from build123d import *

# Parameters (mm, degrees)
BOSS_EXTRUDE1_DEPTH = 20
CUT_EXTRUDE1_DEPTH  = 17
SKETCH3_R           = 2
BOSS_EXTRUDE3_DEPTH = 20


with BuildPart() as part:
    # Sketch1 → Boss-Extrude1 (new body)
    with BuildSketch(Plane.XY):
        with BuildLine():
            Line((-64.955555556, 61.244444444), (75.044444444, 61.244444444))
            ThreePointArc((75.044444444, 61.244444444), (89.186580068, 55.386580068), (95.044444444, 41.244444444))
            Line((95.044444444, 41.244444444), (95.044444444, -48.755555556))
            ThreePointArc((95.044444444, -48.755555556), (89.186580068, -62.897691179), (75.044444444, -68.755555556))
            Line((75.044444444, -68.755555556), (-64.955555556, -68.755555556))
            ThreePointArc((-64.955555556, -68.755555556), (-79.097691179, -62.897691179), (-84.955555556, -48.755555556))
            Line((-84.955555556, -48.755555556), (-84.955555556, 41.244444444))
            ThreePointArc((-84.955555556, 41.244444444), (-79.097691179, 55.386580068), (-64.955555556, 61.244444444))
        make_face()
    extrude(amount=BOSS_EXTRUDE1_DEPTH)

    # Sketch2 → Cut-Extrude1 (cut)
    with BuildSketch(Plane.XY.offset(20)):
        with BuildLine():
            Line((-69.955555556, 56.244444444), (80.044444444, 56.244444444))
            ThreePointArc((80.044444444, 56.244444444), (87.115512256, 53.315512256), (90.044444444, 46.244444444))
            Line((90.044444444, 46.244444444), (90.044444444, -53.755555556))
            ThreePointArc((90.044444444, -53.755555556), (87.115512256, -60.826623367), (80.044444444, -63.755555556))
            Line((80.044444444, -63.755555556), (-69.955555556, -63.755555556))
            ThreePointArc((-69.955555556, -63.755555556), (-77.026623367, -60.826623367), (-79.955555556, -53.755555556))
            Line((-79.955555556, -53.755555556), (-79.955555556, 46.244444444))
            ThreePointArc((-79.955555556, 46.244444444), (-77.026623367, 53.315512256), (-69.955555556, 56.244444444))
        make_face()
    extrude(amount=-CUT_EXTRUDE1_DEPTH, mode=Mode.SUBTRACT)

    # Sketch3 → Boss-Extrude3 (add)
    with BuildSketch(Plane.XY.offset(20)):
        with Locations((-82.455555556, 38.244444444)):
            Circle(SKETCH3_R)
        with Locations((-82.455555556, -45.755555556)):
            Circle(SKETCH3_R)
        with Locations((92.544444444, -45.755555556)):
            Circle(SKETCH3_R)
        with Locations((92.544444444, 38.244444444)):
            Circle(SKETCH3_R)
    extrude(amount=BOSS_EXTRUDE3_DEPTH)


solid = part.part
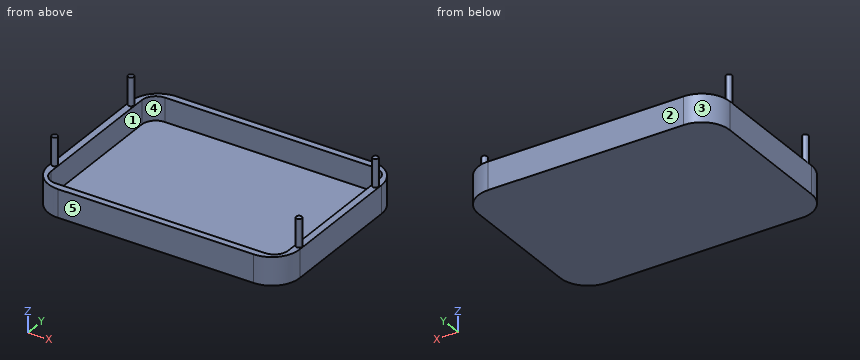
Could you check a few things on this model? Use its own coordinates, in mm. Face numbers are marked on the shaded views. A direction names the side the tool comes from. Coordinates: 2 decimals unless noted, no trailing zeros. Order: outer loops, then holes, each group sorted by start corner. A loop starts at its lowest first (then second) coordinate and runs counter-clockwise, first axis right, second up. Notation, with made-up numbers: (84.25, 60) - (117.25, 60) arc R13 cw to (117.25, 68) - close; hole circle Ø6 at (28.5, 77). An arc over 180 degrees is marked (long way). Answer in a Markdown table with one row per item. Add a question column.
(1) If we mould it in two halves opening along X, with no side actions, what happens to the marked faces 3, 4 and 5? For each: released by +X, released by -X, zero draft, split by the parting line, or undercut.
(2) On a 3-axis mill with a long thin cutter (end or side, diameter ignored), from which of +Z, -Z, +X, -X, +Y, -Y can I reach the whole of each face in a straight line? I mean the marked faces 1 and 2. Say none if no direction works.
(3) If we section it at D-D, the plane z = 34: Please give me the cut outline in (x, y).
(4) If we section it at C-C, the plane y = 8.5: Please give me the cut outline in (x, z).
(5) Will these pins go through, and if not, where does the flat tip stop? pin 1 (3 mm diameter, centred on x = -8.5, y = 39, fed in from +Z); pin 2 (12 mm diameter, centred on y = -49, z = 26.5, fed in from +X).
(6) If we section it at B-B, the plane x = 50: Please give me the cut outline in (y, z), then the cut area to 3 significant figures.
(7) I need wall thicknesses on L1, parallel to X at y = -31, z = 6; L2, parallel to Y at x = 50, z = 18; L3, parallel to X at y = -50, z = 10. Which ranges of each line are inside material? Lowest first, please.
(8) If we section it at A-A, the plane z = 8.5: Please give me the cut outline in (x, y).
Results are:
| question | item | result |
|---|---|---|
| 1 | face 3 | released by -X |
| 1 | face 4 | undercut |
| 1 | face 5 | zero draft |
| 2 | face 1 | +Z |
| 2 | face 2 | +Z, -Z, +X, -X, +Y |
| 3 | outline | circle Ø4 at (-82.46, -45.76); circle Ø4 at (-82.46, 38.24); circle Ø4 at (92.54, -45.76); circle Ø4 at (92.54, 38.24) |
| 4 | outline | (-84.96, 0) - (95.04, 0) - (95.04, 20) - (90.04, 20) - (90.04, 3) - (-79.96, 3) - (-79.96, 20) - (-84.96, 20) - close |
| 5 | pin 1 | stops at z = 3 |
| 5 | pin 2 | stops at x = 94.54 |
| 6 | outline | (-68.76, 0) - (61.24, 0) - (61.24, 20) - (56.24, 20) - (56.24, 3) - (-63.76, 3) - (-63.76, 20) - (-68.76, 20) - close |
| 6 | area | 560 mm2 |
| 7 | L1 | x = -84.96 to -79.96, 90.04 to 95.04 |
| 7 | L2 | y = -68.76 to -63.76, 56.24 to 61.24 |
| 7 | L3 | x = -84.92 to -79.96, 90.04 to 95.01 |
| 8 | outline | (-84.96, -48.76) arc R20 ccw to (-64.96, -68.76) - (75.04, -68.76) arc R20 ccw to (95.04, -48.76) - (95.04, 41.24) arc R20 ccw to (75.04, 61.24) - (-64.96, 61.24) arc R20 ccw to (-84.96, 41.24) - close; hole (-79.96, -53.76) arc R10 ccw to (-69.96, -63.76) - (80.04, -63.76) arc R10 ccw to (90.04, -53.76) - (90.04, 46.24) arc R10 ccw to (80.04, 56.24) - (-69.96, 56.24) arc R10 ccw to (-79.96, 46.24) - close |
